Geometry check sheet. Reference: the model listing, model coordinates, mm. Round coordinates to 2 decimals unless told otherwise and drop trailing zeros. Write each loop counter-clockwise with the first axis right and the second up, starting at its lowest first coordinate (ties: lowest second). Pieces come first, ordered by that corner, then holes. Notation, with made-up numbers: (43, 54.25) -> (85, 54.25) arc R26 ccw to (85, 71.25) -> close; hole circle Ø4 at (-32.75, -5.5). An arc over 180 degrees is marked (long way). Return JSON: item names as keys, results as strings. Group by question number.
from build123d import *

# Parameters (mm, degrees)
SKETCH1_R           = 5
BOSS_EXTRUDE1_DEPTH = 300


with BuildPart() as part:
    # Sketch1 → Boss-Extrude1 (new body)
    with BuildSketch(Plane(origin=(0, 0, 0), x_dir=(1, 0, 0), z_dir=(0, 1, 0))):
        with BuildLine():
            Line((4.191872704, 5.606086267), (11.5870568, 13.001270363))
            Line((11.5870568, 13.001270363), (4.001270363, 13.001270363))
            Line((4.001270363, 13.001270363), (4.001270363, 15.001270363))
            Line((4.001270363, 15.001270363), (15.001270363, 15.001270363))
            Line((15.001270363, 15.001270363), (15.001270363, 4.001270363))
            Line((15.001270363, 4.001270363), (13.001270363, 4.001270363))
            Line((13.001270363, 4.001270363), (13.001270363, 11.5870568))
            Line((13.001270363, 11.5870568), (5.606086267, 4.191872704))
            ThreePointArc((5.606086267, 4.191872704), (7, 0), (5.606086267, -4.191872704))
            Line((5.606086267, -4.191872704), (13.001270363, -11.5870568))
            Line((13.001270363, -11.5870568), (13.001270363, -4.001270363))
            Line((13.001270363, -4.001270363), (15.001270363, -4.001270363))
            Line((15.001270363, -4.001270363), (15.001270363, -15.001270363))
            Line((15.001270363, -15.001270363), (4.001270363, -15.001270363))
            Line((4.001270363, -15.001270363), (4.001270363, -13.001270363))
            Line((4.001270363, -13.001270363), (11.5870568, -13.001270363))
            Line((11.5870568, -13.001270363), (4.191872704, -5.606086267))
            ThreePointArc((4.191872704, -5.606086267), (0, -7), (-4.191872704, -5.606086267))
            Line((-4.191872704, -5.606086267), (-11.5870568, -13.001270363))
            Line((-11.5870568, -13.001270363), (-4.001270363, -13.001270363))
            Line((-4.001270363, -13.001270363), (-4.001270363, -15.001270363))
            Line((-4.001270363, -15.001270363), (-15.001270363, -15.001270363))
            Line((-15.001270363, -15.001270363), (-15.001270363, -4.001270363))
            Line((-15.001270363, -4.001270363), (-13.001270363, -4.001270363))
            Line((-13.001270363, -4.001270363), (-13.001270363, -11.5870568))
            Line((-13.001270363, -11.5870568), (-5.606086267, -4.191872704))
            ThreePointArc((-5.606086267, -4.191872704), (-7, 0), (-5.606086267, 4.191872704))
            Line((-5.606086267, 4.191872704), (-13.001270363, 11.5870568))
            Line((-13.001270363, 11.5870568), (-13.001270363, 4.001270363))
            Line((-13.001270363, 4.001270363), (-15.001270363, 4.001270363))
            Line((-15.001270363, 4.001270363), (-15.001270363, 15.001270363))
            Line((-15.001270363, 15.001270363), (-4.001270363, 15.001270363))
            Line((-4.001270363, 15.001270363), (-4.001270363, 13.001270363))
            Line((-4.001270363, 13.001270363), (-11.5870568, 13.001270363))
            Line((-11.5870568, 13.001270363), (-4.191872704, 5.606086267))
            ThreePointArc((-4.191872704, 5.606086267), (0, 7), (4.191872704, 5.606086267))
        make_face()
        with Locations(Location((0, 0, 0), (0, 0, 270))):
            Circle(SKETCH1_R, mode=Mode.SUBTRACT)
    extrude(amount=BOSS_EXTRUDE1_DEPTH)


solid = part.part
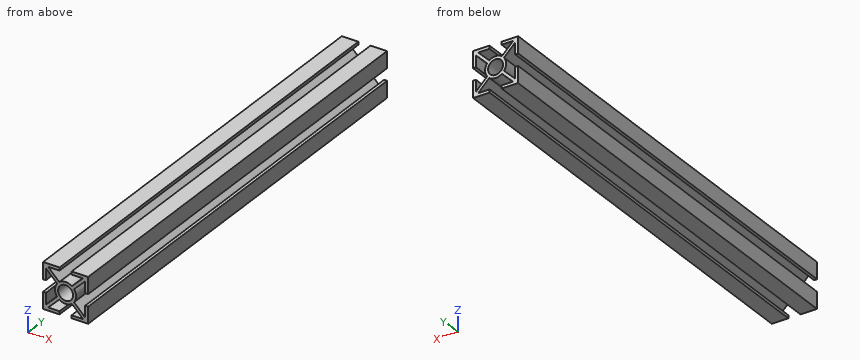
1) Go/stop test with flat-tipped pins: P1, Ø6, axis at x = 0, z = 0, coming from the +Y side; P2, Ø1.5, axis at x = 0.5, y = 194, coming from the -Z side; P3, Ø1, axis at y = 94.5, z = 0, coming from the -X side. Record where each tip stops, or that it passes through.
2) Sectioned sample at A-A on z = 0. Enter the section's corners in (x, y), and give its area (3 significant figures).
3) Sectioned sample at B-B on x = 0. Enter the section's corners in (y, z).
4) Material ranges on probe 1 along X at (y, z) = (67, 0); probe 2 along X at (y, z) = (170, -11); probe 3 along X at (y, z) = (183, 10), recorded low to high. Write a range as [from, to].
Evaluation:
{
 "1": {"P1": "passes through", "P2": "stops at z = -7", "P3": "stops at x = -7"},
 "2": {"outline": "(-7, 0) -> (-5, 0) -> (-5, 300) -> (-7, 300) -> close; (5, 0) -> (7, 0) -> (7, 300) -> (5, 300) -> close", "area": "1,200 mm2"},
 "3": {"outline": "(0, -7) -> (300, -7) -> (300, -5) -> (0, -5) -> close; (0, 5) -> (300, 5) -> (300, 7) -> (0, 7) -> close"},
 "4": {"probe 1": "x = [-7, -5], [5, 7]", "probe 2": "x = [-15, -13], [-12.41, -9.59], [9.59, 12.41], [13, 15]", "probe 3": "x = [-15, -13], [-11.41, -8.59], [8.59, 11.41], [13, 15]"}
}
